Geometry check sheet. Reference: drawing and pictorial views, mm from the part's lowest x, y, z. A direction names the side the tool comes from. Coordinates: 2 decimals unless noted, no trailing zeros. Loops run counter-clockwise (first coordinate to the right, second up) from the corner with the lowest first, then second, coordinate; pieces in that order, holes last. Notation, with made-up numbers: (54, 79) -> (94, 79) arc R34 ccw to (94, 113) -> close; hole circle Ø4 at (-3.5, -33). An arc over 180 degrees is marked (long way). Use one line per item in the form item = value.
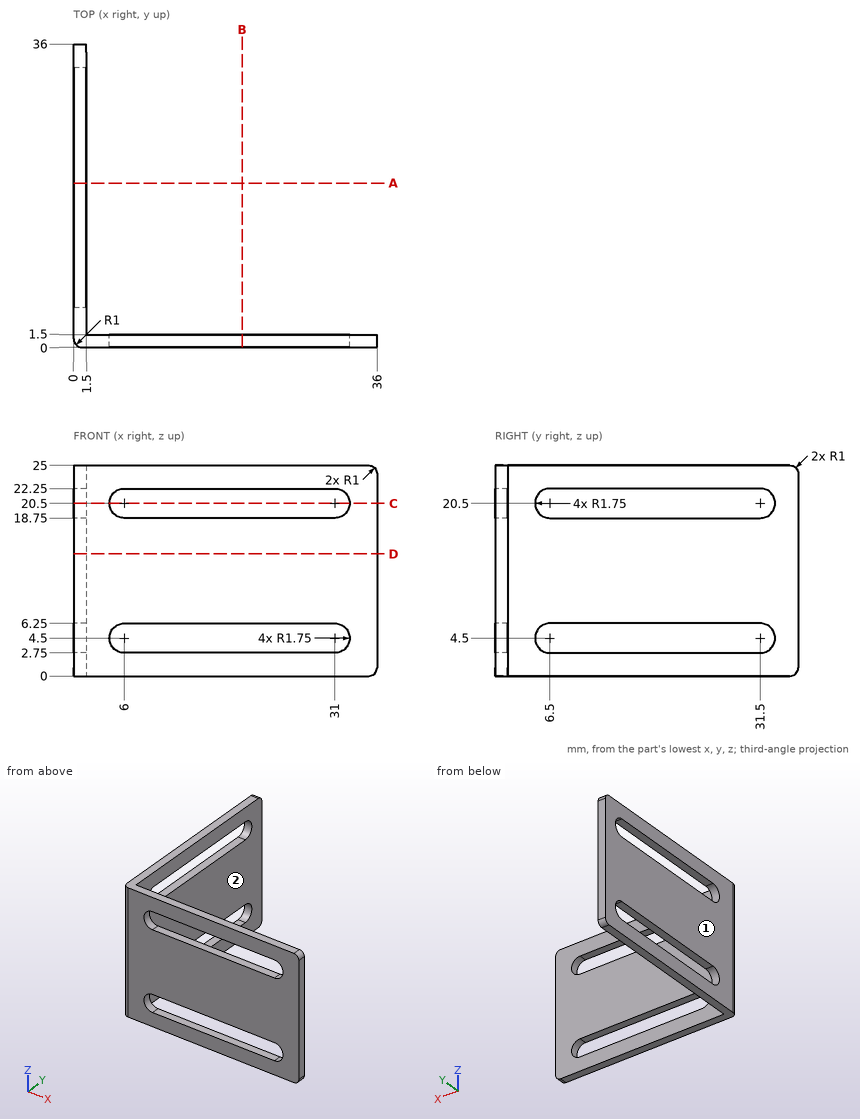
(1) Scan line: line 1 along X through (y, z) = (9, 15). Record every from-to range of solid material in increasing order.
Established:
line_1 = 0 to 1.5
(2) Go/stop test with flat-tipped pins: P1, Ø12, axis at x = 20, z = 17, coming from the +Y side; P2, Ø7.5, axis at y = 20.5, z = 14.5, coming from the +X side. Record where each tip stops, or that it passes through.
Established:
P1 = 1.5
P2 = 1.5
(3) Tool access check on the marked faces 1 and 2. Record the directions out of +Z, -Z, +X, -X, +Y, -Y that give a thin tool (end or side, any length) a straight path to the whole face; none if there is none.
Established:
face_1 = +Z, -Z, -X, +Y, -Y
face_2 = +Z, -Z, +X, +Y
(4) Section check D-D, the plane z = 14.5. Record the boundary of the cut face in (x, y).
Established:
outline = (0, 1) arc R1 ccw to (1, 0) -> (36, 0) -> (36, 1.5) -> (1.5, 1.5) -> (1.5, 36) -> (0, 36) -> close
(5) Section check C-C, the plane z = 20.5. Record the boundary of the cut face in (x, y).
Established:
outline = (0, 1) arc R1 ccw to (1, 0) -> (4.25, 0) -> (4.25, 1.5) -> (1.5, 1.5) -> (1.5, 4.75) -> (0, 4.75) -> close; (0, 33.25) -> (1.5, 33.25) -> (1.5, 36) -> (0, 36) -> close; (32.75, 0) -> (36, 0) -> (36, 1.5) -> (32.75, 1.5) -> close
(6) Section check A-A, the plane y = 19.5. Record the boundary of the cut face in (x, z), plus the area to 3 significant figures.
Established:
outline = (0, 0) -> (1.5, 0) -> (1.5, 2.75) -> (0, 2.75) -> close; (0, 6.25) -> (1.5, 6.25) -> (1.5, 18.75) -> (0, 18.75) -> close; (0, 22.25) -> (1.5, 22.25) -> (1.5, 25) -> (0, 25) -> close
area = 27.0 mm²
